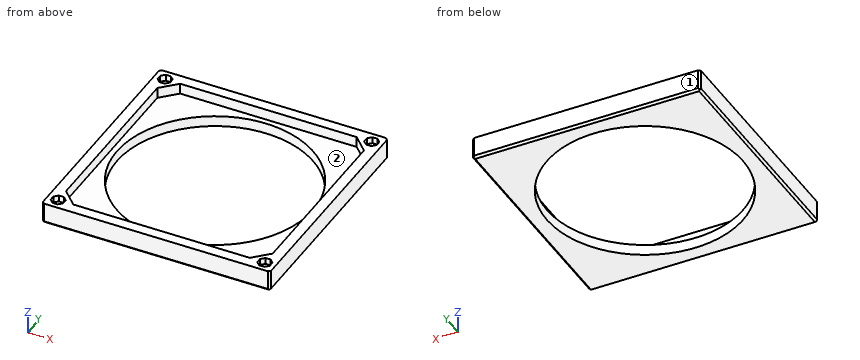
from build123d import *

# Parameters (mm, degrees)
SKETCH1_LARGER_DIA_W  = 106
SKETCH1_LARGER_DIA_H  = 106
BOSS_EXTRUDE1_DEPTH   = 5
SKETCH5_SMALLER_DIA_W = 106
SKETCH5_SMALLER_DIA_H = 106
SKETCH5_SMALLER_DIA_R = 45.5
BOSS_EXTRUDE2_DEPTH   = 5
CUT_EXTRUDE1_DEPTH    = 3
CHAMFER2_SIZE         = 1
CHAMFER3_SIZE         = 1


with BuildPart() as part:
    # Sketch1 larger dia → Boss-Extrude1 (new body)
    with BuildSketch(Plane.XY):
        Rectangle(SKETCH1_LARGER_DIA_W, SKETCH1_LARGER_DIA_H)
        Polygon((-41, 48), (41, 48), (48, 41), (48, -41), (41, -48), (-41, -48), (-48, -41), (-48, 41), align=None, mode=Mode.SUBTRACT)
    extrude(amount=BOSS_EXTRUDE1_DEPTH)

    # Sketch5 smaller dia → Boss-Extrude2 (add)
    with BuildSketch(Plane(origin=(0, 0, 0), x_dir=(-1, 0, 0), z_dir=(0, 0, -1))):
        Rectangle(SKETCH5_SMALLER_DIA_W, SKETCH5_SMALLER_DIA_H)
        Circle(SKETCH5_SMALLER_DIA_R, mode=Mode.SUBTRACT)
    extrude(amount=BOSS_EXTRUDE2_DEPTH)

    # Sketch1 → Cut-Extrude1 (cut)
    with BuildSketch(Plane.XY.offset(5)):
        Polygon((-45.1, 46.798780669), (-45.1, 49.201219331), (-46.798780669, 50.9), (-49.201219331, 50.9), (-50.9, 49.201219331), (-50.9, 46.798780669), (-49.201219331, 45.1), (-46.798780669, 45.1), align=None)
        Polygon((-46.798780669, -45.1), (-45.1, -46.798780669), (-45.1, -49.201219331), (-46.798780669, -50.9), (-49.201219331, -50.9), (-50.9, -49.201219331), (-50.9, -46.798780669), (-49.201219331, -45.1), align=None)
        Polygon((46.798780669, 45.1), (45.1, 46.798780669), (45.1, 49.201219331), (46.798780669, 50.9), (49.201219331, 50.9), (50.9, 49.201219331), (50.9, 46.798780669), (49.201219331, 45.1), align=None)
        Polygon((45.1, -46.798780669), (45.1, -49.201219331), (46.798780669, -50.9), (49.201219331, -50.9), (50.9, -49.201219331), (50.9, -46.798780669), (49.201219331, -45.1), (46.798780669, -45.1), align=None)
    extrude(amount=-CUT_EXTRUDE1_DEPTH, mode=Mode.SUBTRACT)

    # Chamfer2
    chamfer2_edges = [part.edges().sort_by_distance(p)[0] for p in [
        (53, 0, -5),
        (0, -53, -5),
        (-53, 0, -5),
        (0, 53, -5),
    ]]
    chamfer(chamfer2_edges, length=CHAMFER2_SIZE)

    # Chamfer3
    chamfer3_edges = [part.edges().sort_by_distance(p)[0] for p in [
        (-53, 53, 0.5),
        (53, 53, 0.5),
        (53, -53, 0.5),
        (-53, -53, 0.5),
    ]]
    chamfer(chamfer3_edges, length=CHAMFER3_SIZE)


solid = part.part
Verification items for the finished model (mm, model axes). Face numbers are marked on the shaded views. Coordinates: 2 decimals unless noted, no trailing zeros. Order: outer loops, then holes, each group sorted by start corner. A loop starts at its lowest first (then second) coordinate and runs counter-clockwise, first axis right, second up. Notation, with made-up numbers: M 5.5,63 L 48.5,63 A24 cw 48.5,92 Z; hole C 18.25,0.5 d2. An arc over 180 degrees is marked long. One line per item, written item: value. Start each with the question number.
Item 1: Sectioned sample at A-A (y = 0). Enter the section's corners in (x, z).
Item 2: Mould release check, pull along X, two halves, no side actions. Record for the marked faces 1 and 2: released by +X, released by -X, zero draft, split by the parting line, or undercut.
Item 3: Sectioned sample at D-D (z = 3.5). Count the separate pieces of the cut face and the enclosed holes in it, then the cut area to 3 significant figures.
Item 4: Scan lines: probe 1 along X at (y, z) = (-10.5, 4.5); probe 2 along Y at (x, z) = (0, -4). Record each from-to range of solid material in increasing order.
Item 5: Sectioned sample at C-C (z = -2.75). Enter the section's corners in (x, y), then the cut area to 3 significant figures.
Conclusion:
1. outline: M -53,-4 L -52,-5 L -45.5,-5 L -45.5,0 L -48,0 L -48,5 L -53,5 Z; M 45.5,-5 L 52,-5 L 53,-4 L 53,5 L 48,5 L 48,0 L 45.5,0 Z
2. face 1: zero draft
2. face 2: undercut
3. separate pieces: 1
3. enclosed holes: 5
3. area: 2,000 mm^2
4. probe 1: x = -53 to -48, 48 to 53
4. probe 2: y = -53 to -45.5, 45.5 to 53
5. outline: M -53,-52 L -52,-53 L 52,-53 L 53,-52 L 53,52 L 52,53 L -52,53 L -53,52 Z; hole C 0,0 d91
5. area: 4,730 mm^2
